Build history of the part. All positions in model axes, mm. Face numbers are marked on the shaded views. A direction names the side the tool comes from. Coordinates: 2 decimals unless noted, no trailing zeros. Order: outer loops, then holes, each group sorted by start corner. A loop starts at its lowest first (then second) coordinate and runs counter-clockwise, first axis right, second up. Notation, with made-up numbers: (-28.75, -9) - (11.25, -9) arc R19 cw to (11.25, 12) - close; hole circle Ø4 at (-16, 73). An arc over 180 degrees is marked (long way). Write each question's results on one line, items separated by ' | '.
from build123d import *

# Parameters (mm, degrees)
SKETCH_1_W          = 67
SKETCH_1_H          = 40
EXTRUDE_1_DEPTH     = 1
SKETCH_2_W          = 44
SKETCH_2_H          = 2
EXTRUDE_2_DEPTH     = 8.5
SKETCH_3_W          = 45
SKETCH_3_H          = 18.1
EXTRUDE_3_DEPTH     = 5
SKETCH_4_R          = 2.75
CUT_EXTRUDE_1_DEPTH = 5
SKETCH_5_W          = 12
SKETCH_5_H          = 6
EXTRUDE_4_DEPTH     = 7


with BuildPart() as part:
    # ｽｹｯﾁ1 → ﾎﾞｽ - 押し出し1 (new body)
    with BuildSketch(Plane.XY):
        Rectangle(SKETCH_1_W, SKETCH_1_H)
    extrude(amount=EXTRUDE_1_DEPTH)

    # ｽｹｯﾁ2 → ﾎﾞｽ - 押し出し2 (add)
    with BuildSketch(Plane.XY.offset(1)):
        with Locations((0, -1)):
            Rectangle(SKETCH_2_W, SKETCH_2_H)
        with Locations((0, -17)):
            Rectangle(SKETCH_2_W, SKETCH_2_H)
    extrude(amount=EXTRUDE_2_DEPTH)

    # ｽｹｯﾁ3 → ﾎﾞｽ - 押し出し3 (add)
    with BuildSketch(Plane.XY.offset(9.5)):
        with Locations((0, -9)):
            Rectangle(SKETCH_3_W, SKETCH_3_H)
    extrude(amount=EXTRUDE_3_DEPTH)

    # ｽｹｯﾁ4 → ｶｯﾄ - 押し出し1 (cut)
    with BuildSketch(Plane.XY.offset(1)):
        with Locations((-29, -8)):
            Circle(SKETCH_4_R)
        with Locations((29, -8)):
            Circle(SKETCH_4_R)
    extrude(amount=-CUT_EXTRUDE_1_DEPTH, mode=Mode.SUBTRACT)

    # ｽｹｯﾁ5 → ﾎﾞｽ - 押し出し4 (add)
    with BuildSketch(Plane.XY.offset(1)):
        with Locations((-17.5, 10)):
            Rectangle(SKETCH_5_W, SKETCH_5_H)
        with Locations((17.5, 10)):
            Rectangle(SKETCH_5_W, SKETCH_5_H)
    extrude(amount=EXTRUDE_4_DEPTH)


solid = part.part
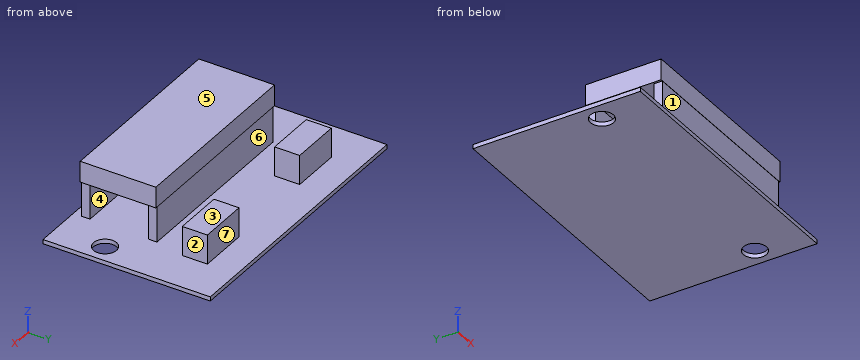
1. Drop flat-ended pins along their axis: pin 1 Ø0.6 at (y, z) = (-1, 4) entering from +X; pin 2 Ø1.8 at (x, y) = (-16.5, 11.5) entering from +Z; pin 3 Ø5 at (x, z) = (-16.5, 9.5) entering from -Y; pin 4 Ø1.5 at (y, z) = (-5, 8.5) entering from +X. Give the stop position or say it passes through.
Solved:
pin 1: stops at x = 22 | pin 2: stops at z = 8 | pin 3: stops at y = -18.05 | pin 4: passes through
2. Band-saw the part on A-A on y = -8. Give the cut face in (x, z), then the cut area to 3 significant figures.
Solved:
outline: (-33.5, 0) - (-31.75, 0) - (-31.75, 1) - (-33.5, 1) - close; (-26.25, 0) - (26.25, 0) - (26.25, 1) - (-26.25, 1) - close; (-22.5, 9.5) - (22.5, 9.5) - (22.5, 14.5) - (-22.5, 14.5) - close; (31.75, 0) - (33.5, 0) - (33.5, 1) - (31.75, 1) - close | area: 281 mm2
3. Band-saw the part on C-C on z = 7. Give the cut face in (x, y), then the cut area to 3 significant figures.
Solved:
outline: (-23.5, 7) - (-11.5, 7) - (-11.5, 13) - (-23.5, 13) - close; (-22, -18) - (22, -18) - (22, -16) - (-22, -16) - close; (-22, -2) - (22, -2) - (22, 0) - (-22, 0) - close; (11.5, 7) - (23.5, 7) - (23.5, 13) - (11.5, 13) - close | area: 320 mm2
4. Two-plate mould, pull along Z, no slides. Class the marked faces 4, 5, 6 and 7: +Z half, -Z half, draft (parallel to the pull), parting line (faces both ways), or undercut.
Solved:
face 4: undercut | face 5: +Z half | face 6: undercut | face 7: draft
5. Band-saw the part on B-B on x = -20.5. Give the cut face in (y, z).
Solved:
outline: (-20, 0) - (20, 0) - (20, 1) - (13, 1) - (13, 8) - (7, 8) - (7, 1) - (0, 1) - (0, 9.5) - (0.05, 9.5) - (0.05, 14.5) - (-18.05, 14.5) - (-18.05, 9.5) - (-18, 9.5) - (-18, 1) - (-20, 1) - close; hole (-16, 1) - (-2, 1) - (-2, 9.5) - (-16, 9.5) - close
6. Tool access for the marked faces 1, 2 and 3: list every direction of +Z, -Z, +X, -X, +Y, -Y with a clear straight run to the whole face (end or side of a thin tool).
Solved:
face 1: +X, -X, -Y | face 2: +Z, +X, +Y, -Y | face 3: +Z, +X, -X, +Y
7. Band-saw the part on D-D on x = 29. Give the cut face in (y, z), then the cut area to 3 significant figures.
Solved:
outline: (-20, 0) - (-10.75, 0) - (-10.75, 1) - (-20, 1) - close; (-5.25, 0) - (20, 0) - (20, 1) - (-5.25, 1) - close | area: 34.5 mm2
8. Probe line 1 (Y direction, x = 19.5, z = 3); line 2 (Z direction, x = 2, y = -4.5); line 3 (Y direction, x = -29, z = 0.65). List the from-to ranges inside material, lowest first.
Solved:
line 1: y = -18 to -16, -2 to 0, 7 to 13 | line 2: z = 0 to 1, 9.5 to 14.5 | line 3: y = -20 to -10.75, -5.25 to 20
